Design review of the part shown in the three views and the two pictorial views. Dimensions are in mm from the part's minimum x, y and z. A direction names the side the tool comes from. Round coordinates to 2 decimals unless told otherwise and drop trailing zeros. Write each loop counter-clockwise with the first axis right and the second up, starting at its lowest first coordinate (ties: lowest second). Pieces come first, ordered by that corner, then holes. Notation, with made-up numbers: (75.25, -21) - (110.25, -21) arc R24 cw to (110.25, 9) - close; hole circle Ø10 at (17.25, 71). An arc over 180 degrees is marked (long way). One line per item, written item: value. Start each with the question number.
Q1. Add section C-C on x = 3.5. Write out the cut boundary in (y, z), and give its area (3 significant figures).
Q2. Clearance check with flat-ended pins moving along their axes: pin 1 Ø6.5 at (x, y) = (2, 5) entering from +Z; pin 2 Ø1 at (y, z) = (18, 10) entering from -X; pin 3 Ø1.5 at (y, z) = (13.5, 11) entering from +X; pin 4 Ø1.7 at (x, y) = (36, 4) entering from +Z. State where each tip first meets the part, or that it passes through.
Q3. Tool access review of the marked faces 1, 2, 3 and 4: name each direction out of +Z, -Z, +X, -X, +Y, -Y from which nothing blocks a thin tool from reaching the whole face with its end or side.
Q4. Add section B-B on y = 26. Write out the cut boundary in (x, z).
Q5. Add section D-D on x = 17. Write out the cut boundary in (y, z), and give its area (3 significant figures).
Q6. Add section A-A on z = 16. Write out the cut boundary in (x, y), and give its area (3 significant figures).
Q7. Mouldability with a two-part tool opening along Y and no side actions: class the marked faces 5, 6 and 7 as +Y half, -Y half, draft (parallel to the pull), parting line (faces both ways), or undercut.
Q8. For probe 1 along Y at (x, z) = (4, 0.75); probe 2 along X at (y, z) = (37.5, 16); probe 3 along Y at (x, z) = (33, 13.25), list the stretches that pass through material, from the lowest coordinate up.
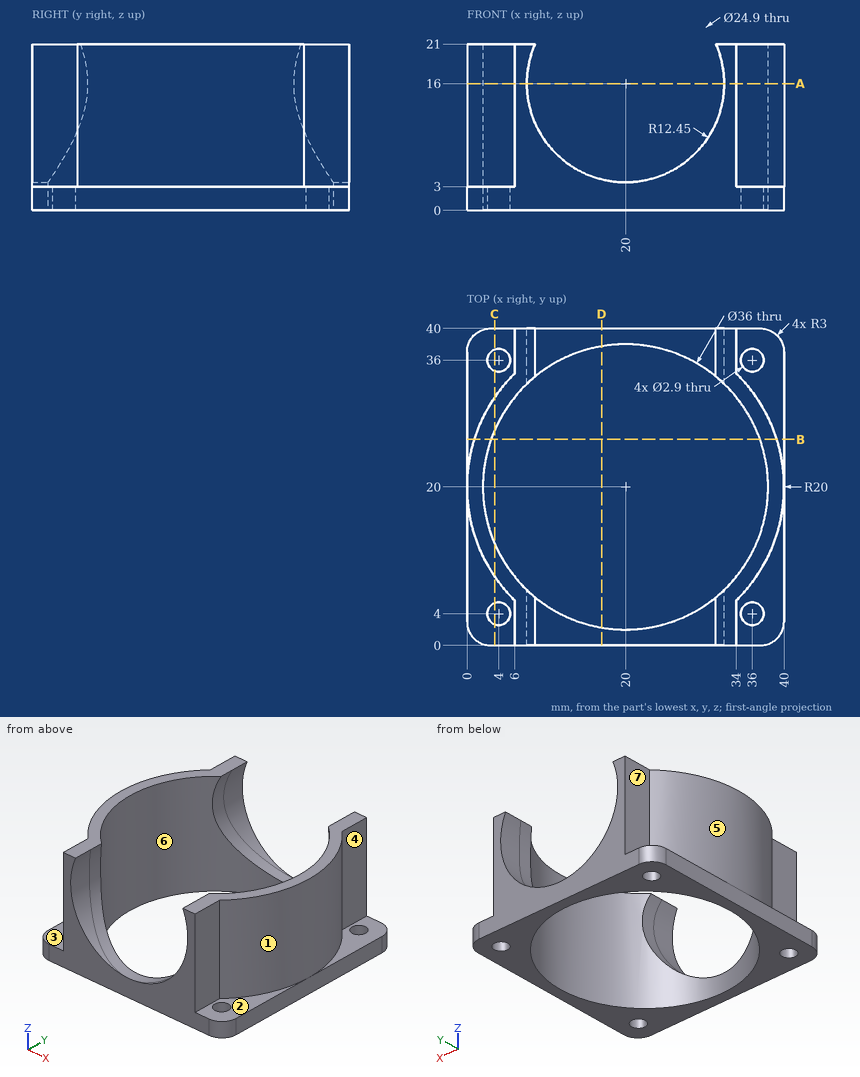
Result set:
1. outline: (0, 0) - (2.64, 0) - (2.64, 3) - (0, 3) - close; (5.36, 0) - (12.81, 0) - (12.81, 21) - (8.7, 21) - (8.7, 3) - (5.36, 3) - close; (27.19, 0) - (34.64, 0) - (34.64, 3) - (31.3, 3) - (31.3, 21) - (27.19, 21) - close; (37.36, 0) - (40, 0) - (40, 3) - (37.36, 3) - close
1. area: 208 mm^2
2. pin 1: stops at z = 3
2. pin 2: stops at x = 0.06
2. pin 3: stops at x = 39.16
2. pin 4: passes through
3. face 1: +Z, +X
3. face 2: +Z, +X, -Y
3. face 3: +Z, -X, -Y
3. face 4: +Z, +X, +Y
4. outline: (0, 0) - (3.03, 0) - (3.03, 21) - (0.92, 21) - (0.92, 3) - (0, 3) - close; (36.97, 0) - (40, 0) - (40, 3) - (39.08, 3) - (39.08, 21) - (36.97, 21) - close
5. outline: (0, 0) - (2.25, 0) - (2.25, 3.92) - (0, 3.92) - close; (37.75, 0) - (40, 0) - (40, 3.92) - (37.75, 3.92) - close
5. area: 17.6 mm^2
6. outline: (6, 0) - (7.55, 0) - (7.55, 7) arc R18 cw to (7.55, 33) - (7.55, 40) - (6, 40) - (6, 34.28) arc R20 ccw to (6, 5.72) - close; (32.45, 0) - (34, 0) - (34, 5.72) arc R20 ccw to (34, 34.28) - (34, 40) - (32.45, 40) - (32.45, 33) arc R18 cw to (32.45, 7) - close
6. area: 161 mm^2
7. face 5: parting line
7. face 6: undercut
7. face 7: draft
8. probe 1: y = 0 to 2.55, 5.45 to 11.75, 28.25 to 34.55, 37.45 to 40
8. probe 2: x = 6 to 7.55, 32.45 to 34
8. probe 3: y = 0 to 7.55, 32.45 to 40
